Source: CAD feature listing. Evaluate the final solid. Frame: model axes, mm. Round coordinates to 2 decimals unless told otherwise and drop trailing zeros. Write each loop counter-clockwise with the first axis right and the second up, starting at its lowest first coordinate (ties: lowest second). Pieces come first, ordered by that corner, then holes. Notation, with made-up numbers: M 87,49 L 139,49 A20 cw 139,75 Z; hole C 35,46 d6. An arc over 180 degrees is marked long. Answer in a Markdown table with one row per item. Add a question column.
Item 1: Mould query, pull axis Y, two halves, no side actions, for faces 1 (the face through (0.86, -17.95, 0.99)), 2 (the face through (-5.961, 26.846, 0.493)), 3 (the face through (0, 0, 0)), 4 (the face through (-13.68, 0.49, 0.99)). Classes: released by +Y, released by -Y, zero draft, split by the parting line, or undercut.
Item 2: Cut plane A-A on y = 0. Return loops of the section in (x, z).
Item 3: Cut plane C-C on z = 1.55. Return loops of the section in (x, y) (3 decimals).
Item 4: Material intervals for probe 1 along Y at (x, z) = (0, 1.4); probe 2 along Y at (x, z) = (0, 1.2); probe 3 along X at (y, z) = (14.5, 1.2), sorted ascending.
Item 5: Contact query for flat-ended pins moving along their axis: pin 1 (3.5 mm diameter, centred on x = 15.875, y = 0, fed in from -Z); pin 2 (1 mm diameter, centred on y = -10.5, z = 1, fed in from +X). Output: stop coordinate, or through.
Autodesk Inventor part; units mm, degrees
ref_plane "YZ Plane" through (0, 0, 0) normal (1, 0, 0) x (0, 1, 0)
ref_plane "XZ Plane" through (0, 0, 0) normal (0, 1, 0) x (-1, 0, 0)
ref_plane "XY Plane" through (0, 0, 0) normal (0, 0, 1) x (1, 0, 0)
sketch "Sketch1" plane through (0, 0, 0) normal (0, 0, 1) x (1, 0, 0)
  circle A0 centre (0, 0) radius 27.5
  dimension "d0" = 55
extrude "Extrusion1" add sketch "Sketch1" along normal blind 2
chamfer "Chamfer1" distance 1 angle 45 1 edges at (-27.5, 0, 2)
sketch "Sketch2" plane through (0, 0, 2) normal (0, 0, 1) x (1, 0, 0)
  circle A0 centre (0, 0) radius 15.875 construction
  point P0 (0, 15.875)
  point P1 (-15.875, 0)
  point P2 (0, -15.875)
  point P3 (15.875, 0)
  dimension "d6" = 31.75
  dimension "d9" = 360
hole "Hole1" at (0, 15.875, 2) at (-15.875, 0, 2) at (0, -15.875, 2) at (15.875, 0, 2) direction (0, 0, -1) diameter 4.4958 end through all
properties part number "53t_gt2_flange" material "Aluminum 6061"
Results below:
| question | item | result |
|---|---|---|
| 1 | face 1 | undercut |
| 1 | face 2 | split by the parting line |
| 1 | face 3 | zero draft |
| 1 | face 4 | undercut |
| 2 | outline | M -27.5,0 L -18.12,0 L -18.12,2 L -26.5,2 L -27.5,1 Z; M -13.63,0 L 13.63,0 L 13.63,2 L -13.63,2 Z; M 18.12,0 L 27.5,0 L 27.5,1 L 26.5,2 L 18.12,2 Z |
| 3 | outline | C 0,0 d53.9; hole C -15.875,0 d4.496; hole C 0,-15.875 d4.496; hole C 0,15.875 d4.496; hole C 15.875,0 d4.496 |
| 4 | probe 1 | -27.1 to -18.12, -13.63 to 13.63, 18.12 to 27.1 |
| 4 | probe 2 | -27.3 to -18.12, -13.63 to 13.63, 18.12 to 27.3 |
| 4 | probe 3 | -23.13 to -1.78, 1.78 to 23.13 |
| 5 | pin 1 | through |
| 5 | pin 2 | x = 25.62 |
